The model under review builds one solid part; all positions refer to its coordinate system, in mm. A direction names the side the tool comes from. Give positions to 0.01 mm unless a question says otherwise; leave off trailing zeros. Order: outer loops, then holes, each group sorted by start corner. A loop starts at its lowest first (then second) coordinate and runs counter-clockwise, first axis right, second up.
```python
from build123d import *

# Parameters (mm, degrees)
SKETCH_1_R          = 4.5
SKETCH_1_R_2        = 1.25
EXTRUDE_1_DEPTH     = 8.5
EXTRUDE_2_DEPTH     = 12
CHAMFER_1_SIZE      = 2.5
SKETCH_2_R          = 8
CUT_EXTRUDE_1_DEPTH = 6
FILLET_1_R          = 2
FILLET_2_R          = 0.5


with BuildPart() as part:
    # Sketch 1 → Extrude 1 (new body)
    with BuildSketch(Plane(origin=(0, 0, 0), x_dir=(1, 0, 0), z_dir=(0, 1, 0))):
        with BuildLine():
            ThreePointArc((-14.815194903, 21), (-18.172644276, 18.172644276), (-21, 14.815194903))
            Line((-21, 14.815194903), (-21, -14.815194903))
            ThreePointArc((-21, -14.815194903), (-18.172644276, -18.172644276), (-14.815194903, -21))
            Line((-14.815194903, -21), (14.815194903, -21))
            ThreePointArc((14.815194903, -21), (18.172644276, -18.172644276), (21, -14.815194903))
            Line((21, -14.815194903), (21, 14.815194903))
            ThreePointArc((21, 14.815194903), (18.172644276, 18.172644276), (14.815194903, 21))
            Line((14.815194903, 21), (-14.815194903, 21))
        make_face()
        Circle(SKETCH_1_R, mode=Mode.SUBTRACT)
        with Locations((-15.5, 15.5)):
            Circle(SKETCH_1_R_2, mode=Mode.SUBTRACT)
        with Locations((15.5, 15.5)):
            Circle(SKETCH_1_R_2, mode=Mode.SUBTRACT)
        with Locations((15.5, -15.5)):
            Circle(SKETCH_1_R_2, mode=Mode.SUBTRACT)
        with Locations((-15.5, -15.5)):
            Circle(SKETCH_1_R_2, mode=Mode.SUBTRACT)
    extrude(amount=EXTRUDE_1_DEPTH)

    # Sketch 1_4 → Extrude 2 (add)
    with BuildSketch(Plane(origin=(0, 0, 0), x_dir=(1, 0, 0), z_dir=(0, 1, 0))):
        with BuildLine():
            ThreePointArc((21, -14.815194903), (18.172644276, -18.172644276), (14.815194903, -21))
            Line((14.815194903, -21), (17.2, -21))
            Line((17.2, -21), (21, -17.2))
            Line((21, -17.2), (21, -14.815194903))
        make_face()
        with BuildLine():
            ThreePointArc((-14.815194903, -21), (-18.172644276, -18.172644276), (-21, -14.815194903))
            Line((-21, -14.815194903), (-21, -17.2))
            Line((-21, -17.2), (-17.2, -21))
            Line((-17.2, -21), (-14.815194903, -21))
        make_face()
        with BuildLine():
            Line((-17.2, 21), (-21, 17.2))
            Line((-21, 17.2), (-21, 14.815194903))
            ThreePointArc((-21, 14.815194903), (-18.172644276, 18.172644276), (-14.815194903, 21))
            Line((-14.815194903, 21), (-17.2, 21))
        make_face()
        with BuildLine():
            Line((17.2, 21), (14.815194903, 21))
            ThreePointArc((14.815194903, 21), (18.172644276, 18.172644276), (21, 14.815194903))
            Line((21, 14.815194903), (21, 17.2))
            Line((21, 17.2), (17.2, 21))
        make_face()
    extrude(amount=EXTRUDE_2_DEPTH)

    # Chamfer 1
    chamfer_1_edges = [part.edges().sort_by_distance(p)[0] for p in [
        (-16.75, 0, 15.5),
        (14.25, 0, 15.5),
        (14.25, 0, -15.5),
        (-16.75, 0, -15.5),
    ]]
    chamfer(chamfer_1_edges, length=CHAMFER_1_SIZE)

    # Sketch 2 → Cut-Extrude 1 (cut)
    with BuildSketch(Plane(origin=(0, 8.5, 0), x_dir=(1, 0, 0), z_dir=(0, 1, 0))):
        Circle(SKETCH_2_R)
    extrude(amount=-CUT_EXTRUDE_1_DEPTH, mode=Mode.SUBTRACT)

    # Fillet 1
    fillet_1_edges = [part.edges().sort_by_distance(p)[0] for p in [
        (17.2, 6, 21),
        (21, 6, 17.2),
        (-21, 6, 17.2),
        (-17.2, 6, 21),
        (-17.2, 6, -21),
        (-21, 6, -17.2),
        (21, 6, -17.2),
        (17.2, 6, -21),
    ]]
    fillet(fillet_1_edges, radius=FILLET_1_R)

    # Fillet 2
    fillet_2_edges = [part.edges().sort_by_distance(p)[0] for p in [
        (21, 0, 0),
        (0, 0, 21),
        (-19.1, 0, 19.1),
        (-21, 0, 0),
        (-19.1, 0, -19.1),
        (0, 0, -21),
        (19.1, 0, -19.1),
        (19.1, 0, 19.1),
        (20.847759065, 0, -17.13693974),
        (17.13693974, 0, -20.847759065),
        (-17.13693974, 0, -20.847759065),
        (-20.847759065, 0, -17.13693974),
        (-20.847759065, 0, 17.13693974),
        (-17.13693974, 0, 20.847759065),
        (17.13693974, 0, 20.847759065),
        (20.847759065, 0, 17.13693974),
    ]]
    fillet(fillet_2_edges, radius=FILLET_2_R)


solid = part.part
```
Item 1: Clearance check with a flat-ended pin moving along its axis: pin 1 Ø13 at (x, z) = (3.5, 0.5) entering from +Y. State where the tip first meets the part, or that it passes through.
Values found:
pin 1: stops at y = 8.5
Item 2: For faces 1 (the cylindrical face through (18.216, 10.226, 18.129)), 2 (the flat face through (0, 4, -21)), list the 3-axis set-ups (+Z, -Z, +X, -X, +Y, -Y) from which the entire face can be reached by the end or side of a thin tool; tool diameter is ignored.
Values found:
face 1: +Y
face 2: -Z, +X, -X, +Y, -Y
Item 3: Draft analysis for pull direction Z (two halves, no side actions). For faces 3 (the cylindrical face through (20.85, 6.33, -17.13)), 4 (the cylindrical face through (-0.59, 1.23, -4.46)), 5 (the flat face through (21, 4, 0)), state which applies: released by +Z, released by -Z, zero draft, split by the parting line, or undercut.
Values found:
face 3: released by -Z
face 4: undercut
face 5: zero draft
Item 4: Take a section at A-A (x = 0). Give the boundary of the cut face in (y, z).
Values found:
outline: (0, -20.5) arc R0.5 ccw to (0.5, -21) - (8.5, -21) - (8.5, -8) - (2.5, -8) - (2.5, -4.5) - (0, -4.5) - close; (0, 4.5) - (2.5, 4.5) - (2.5, 8) - (8.5, 8) - (8.5, 21) - (0.5, 21) arc R0.5 ccw to (0, 20.5) - close
Item 5: For line 1 (Z direction, x = -15.5, y = 4.9); line 2 (Z direction, x = 0, y = 1.7), list the stretches that pass through material, from the lowest coordinate up.
Values found:
line 1: z = -21 to -16.75, -14.25 to 14.25, 16.75 to 21
line 2: z = -21 to -4.5, 4.5 to 21
Item 6: Take a section at B-B (y = 1). Give the boundary of the cut face in (x, z), and give its area (3 significant figures).
Values found:
outline: (-21, -16.37) arc R2 ccw to (-20.41, -17.79) - (-17.79, -20.41) arc R2 ccw to (-16.37, -21) - (16.37, -21) arc R2 ccw to (17.79, -20.41) - (20.41, -17.79) arc R2 ccw to (21, -16.37) - (21, 16.37) arc R2 ccw to (20.41, 17.79) - (17.79, 20.41) arc R2 ccw to (16.37, 21) - (-16.37, 21) arc R2 ccw to (-17.79, 20.41) - (-20.41, 17.79) arc R2 ccw to (-21, 16.37) - close; hole circle Ø5.5 at (-15.5, -15.5); hole circle Ø5.5 at (-15.5, 15.5); hole circle Ø9 at (0, 0); hole circle Ø5.5 at (15.5, -15.5); hole circle Ø5.5 at (15.5, 15.5)
area: 1,580 mm2
Item 7: Take a section at C-C (z = 0). Give the boundary of the cut face in (x, y).
Values found:
outline: (-21, 0.5) arc R0.5 ccw to (-20.5, 0) - (-4.5, 0) - (-4.5, 2.5) - (-8, 2.5) - (-8, 8.5) - (-21, 8.5) - close; (4.5, 0) - (20.5, 0) arc R0.5 ccw to (21, 0.5) - (21, 8.5) - (8, 8.5) - (8, 2.5) - (4.5, 2.5) - close
Item 8: Take a section at D-D (x = -15.5). Give the boundary of the cut face in (y, z), and give its area (3 significant figures).
Values found:
outline: (0, -20.5) arc R0.5 ccw to (0.5, -21) - (12, -21) - (12, -20.5) - (8.5, -20.5) - (8.5, -16.75) - (2.5, -16.75) - (0, -19.25) - close; (0, -11.75) - (2.5, -14.25) - (8.5, -14.25) - (8.5, 14.25) - (2.5, 14.25) - (0, 11.75) - close; (0, 19.25) - (2.5, 16.75) - (8.5, 16.75) - (8.5, 20.5) - (12, 20.5) - (12, 21) - (0.5, 21) arc R0.5 ccw to (0, 20.5) - close
area: 305 mm2
